from build123d import *

# Parameters (mm, degrees)
F0_W     = 68
F0_H     = 250
F1_DEPTH = 19
F2_W     = 17
F2_H     = 19
F3_DEPTH = 19.001
F4_W     = 17
F4_H     = 19
F5_DEPTH = 19.001


with BuildPart() as f1:
    # F0 (on Front) → F1 (new body)
    with BuildSketch(Plane.XZ):
        Rectangle(F0_W, F0_H)
    extrude(amount=F1_DEPTH)

    # F2 (on face) → F3 (cut, through all)
    with BuildSketch(Plane.XZ.offset(19)):
        with Locations((8.5, 115.5)):
            Rectangle(F2_W, F2_H)
        with Locations((-25.5, 115.5)):
            Rectangle(F2_W, F2_H)
    extrude(amount=-F3_DEPTH, mode=Mode.SUBTRACT)

    # F4 (on face) → F5 (cut, through all)
    with BuildSketch(Plane(origin=(0, 0, 0), x_dir=(-1, 0, 0), z_dir=(0, 1, 0))):
        with Locations((25.5, -115.5)):
            Rectangle(F4_W, F4_H)
        with Locations((-8.5, -115.5)):
            Rectangle(F4_W, F4_H)
    extrude(amount=-F5_DEPTH, mode=Mode.SUBTRACT)


solid = f1.part
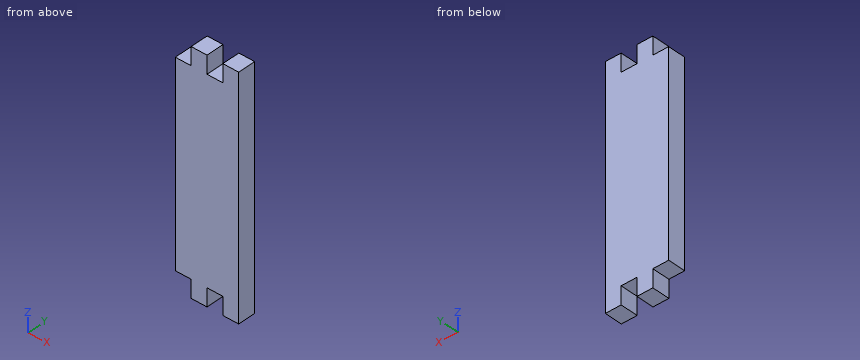
Read the model definition and answer for the solid it produces. Units are mm, in the model's axes. Round coordinates to 2 decimals unless told otherwise and drop trailing zeros. Write each loop counter-clockwise with the first axis right and the second up, starting at its lowest first coordinate (ties: lowest second). Pieces come first, ordered by that corner, then holes. Notation, with made-up numbers: (44.25, 73) - (90.25, 73) arc R3 cw to (90.25, 77) - close; hole circle Ø9 at (37, 47). An arc over 180 degrees is marked (long way). Use a Markdown table: item, result.
(1) The part is cut by section B-B (x = -22.5). Write down the section's boundary in (y, z), then the cut area to 3 significant figures.
Reported:
| item | result |
|---|---|
| outline | (-19, -106) - (0, -106) - (0, 106) - (-19, 106) - close |
| area | 4,030 mm2 |
(2) Each of these flat-tipped pins is pushed along its axis until it touches: pin 1 Ø8.5 at (x, y) = (-23, -13.5) entering from -Z; pin 2 Ø8.5 at (x, y) = (-28.5, -9) entering from +Z; pin 3 Ø9.5 at (y, z) = (-6.5, -118) entering from -X; pin 4 Ø6 at (x, y) = (16.5, -4) entering from +Z. Where does it stop, or does it pass through?
Reported:
| item | result |
|---|---|
| pin 1 | z = -106 |
| pin 2 | z = 106 |
| pin 3 | x = -17 |
| pin 4 | z = 125 |
(3) A straight line is drawn through the part: line 1 along Z through (x, y) = (9.5, -2.75). Find the intervals that lie inside material, in ascending order. Write a range as [from, to].
Reported:
| item | result |
|---|---|
| line 1 | [-106, 106] |
(4) The part is cut by section A-A (y = -5.5). Write down the section's boundary in (x, z).
Reported:
| item | result |
|---|---|
| outline | (-34, -106) - (-17, -106) - (-17, -125) - (0, -125) - (0, -106) - (17, -106) - (17, -125) - (34, -125) - (34, 125) - (17, 125) - (17, 106) - (0, 106) - (0, 125) - (-17, 125) - (-17, 106) - (-34, 106) - close |
